Study the drawing (mm; zero at the part's minimum x, y, z) and answer. Coordinates: 2 decimals unless noted, no trailing zeros. Loops run counter-clockwise (first coordinate to the right, second up) from the corner with the lowest first, then second, coordinate; pieces in that order, holes last. Notation, with made-up numbers: (78.25, -35) - (118.25, -35) arc R24 cw to (118.25, -2) - close; hole circle Ø9 at (63.25, -31.75). An arc over 180 degrees is marked (long way). Use CSV: the item, a comma, the result in double quotes.
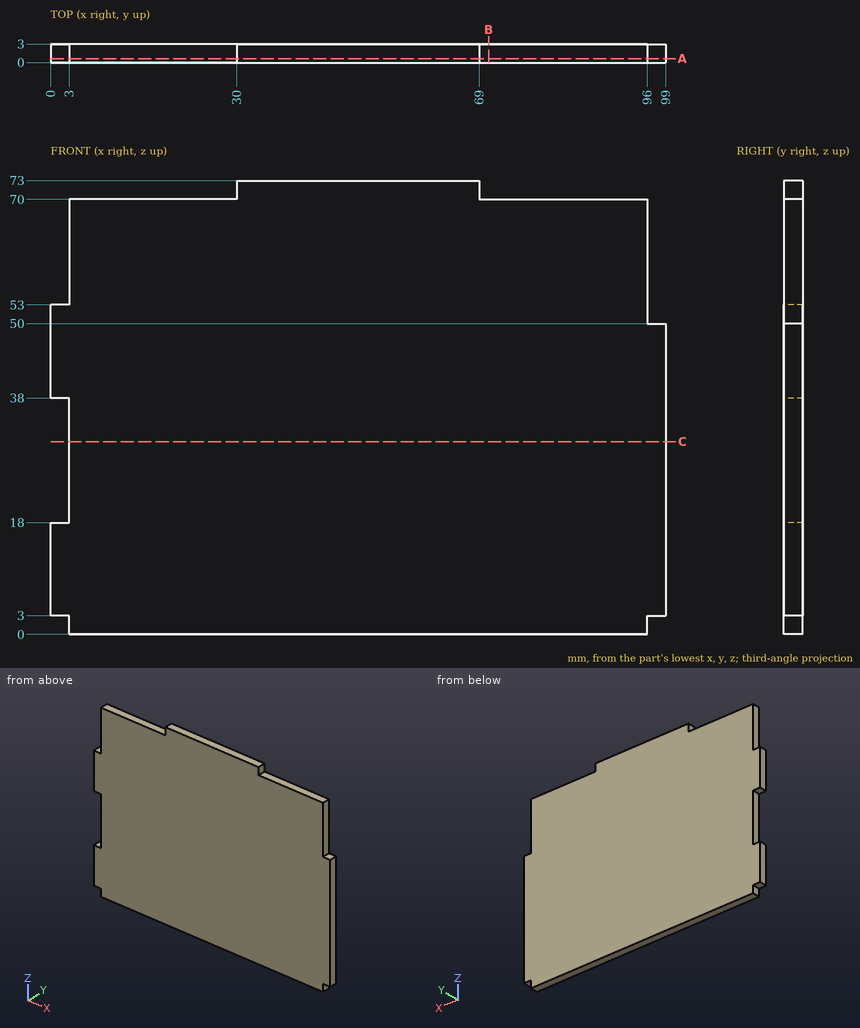
Q1. Given P1, Ø1.5, axis at y = 2, z = 30, coming from the -X side; P2, Ø1.5, axis at x = 11, y = 1.5, coming from the +Z side; P3, Ø1.5, axis at x = 97.5, y = 1.5, coming from the +Z side, each flat-ended and moving along its own axis, determine where each tip first touches the part or whether it passes through.
Reported:
P1,"stops at x = 3"
P2,"stops at z = 70"
P3,"stops at z = 50"
Q2. The part is cut by section A-A on y = 0.65. Determine the outline of the cut face in (x, z), and give its area (3 significant figures).
Reported:
outline,"(0, 3) - (3, 3) - (3, 0) - (96, 0) - (96, 3) - (99, 3) - (99, 50) - (96, 50) - (96, 70) - (69, 70) - (69, 73) - (30, 73) - (30, 70) - (3, 70) - (3, 53) - (0, 53) - (0, 38) - (3, 38) - (3, 18) - (0, 18) - close"
area,"6,860 mm²"
Q3. The part is cut by section B-B on x = 70.5. Determine the outline of the cut face in (y, z).
Reported:
outline,"(0, 0) - (3, 0) - (3, 70) - (0, 70) - close"
Q4. Find the intervals of material crossed by probe 1 along Z at (x, y) = (5, 0.6); probe 2 along X at (y, z) = (1.15, 34.5); probe 3 along X at (y, z) = (0.15, 59), in increasing order. Write a range as [from, to].
Reported:
probe 1,"z = [0, 70]"
probe 2,"x = [3, 99]"
probe 3,"x = [3, 96]"
Q5. The part is cut by section C-C on z = 31. Determine the outline of the cut face in (x, y), and give its area (3 significant figures).
Reported:
outline,"(3, 0) - (99, 0) - (99, 3) - (3, 3) - close"
area,"288 mm²"
